CAD build for the part. Positions are in the model's coordinates, mm. Face numbers are marked on the shaded views. A direction names the side the tool comes from. Give positions to 0.01 mm unless a question says otherwise; leave off trailing zeros. Write each loop counter-clockwise with the first axis right and the second up, starting at its lowest first coordinate (ties: lowest second). Pieces come first, ordered by that corner, then holes. Notation, with made-up numbers: (25, 65) - (60, 65) arc R21 cw to (60, 100) - close; hole circle Ø5 at (-23, 40). An arc over 180 degrees is marked (long way). Answer as a JSON object with one key per item and string values.
from build123d import *

# Parameters (mm, degrees)
F0_R     = 19.05
F0_R_2   = 3.81
F0_R_3   = 5.4991
F1_DEPTH = 6.35
F0_R_4   = 2.7305
F2_DEPTH = 19.05
F4_DEPTH = 2


# Not quite as in the source:
# - a fillet or chamfer that OpenCascade refuses, or shapes differently, is made with other operations: its cross-section is extruded or revolved along the edge and cut away or added


with BuildPart() as f1:
    # F0 (on Top) → F1 (new body)
    with BuildSketch(Plane.XY):
        Circle(F0_R)
        with Locations((-9.6237072996, -5.55625)):
            Circle(F0_R_2, mode=Mode.SUBTRACT)
        with Locations((9.6237072996, -5.55625)):
            Circle(F0_R_2, mode=Mode.SUBTRACT)
        Circle(F0_R_3, mode=Mode.SUBTRACT)
        with Locations((0, 11.1125)):
            Circle(F0_R_2, mode=Mode.SUBTRACT)
    extrude(amount=F1_DEPTH)

    # F0 (on Top) → F2 (join)
    with BuildSketch(Plane.XY):
        Circle(F0_R_3)
        Circle(F0_R_4, mode=Mode.SUBTRACT)
    extrude(amount=F2_DEPTH)

    # F3 (on face) → F4 (cut)
    with BuildSketch(Plane.XY.offset(19.05)):
        with BuildLine():
            Line((1, 2.5407932324), (1, 5.4074116553))
            ThreePointArc((1, 5.4074116553), (0, 5.4991), (-1, 5.4074116553))
            Line((-1, 5.4074116553), (-1, 2.5407932324))
            ThreePointArc((-1, 2.5407932324), (0, 2.7305), (1, 2.5407932324))
        make_face()
        with BuildLine():
            Line((1, -5.4074116553), (1, -2.5407932324))
            ThreePointArc((1, -2.5407932324), (0, -2.7305), (-1, -2.5407932324))
            Line((-1, -2.5407932324), (-1, -5.4074116553))
            ThreePointArc((-1, -5.4074116553), (0, -5.4991), (1, -5.4074116553))
        make_face()
    extrude(amount=-F4_DEPTH, mode=Mode.SUBTRACT)

    # F5: chamfer of 4.445 on 1 edges, made by hand

    # F5_s1 → F5_t2 (revolve, cut)
    with BuildSketch(Plane.XZ):
        Polygon((19.05, 4.445), (14.605, 0), (19.05, 0), align=None)
    revolve(axis=Axis((0, 0, 0), (0, 0, 1)), mode=Mode.SUBTRACT)


solid = f1.part
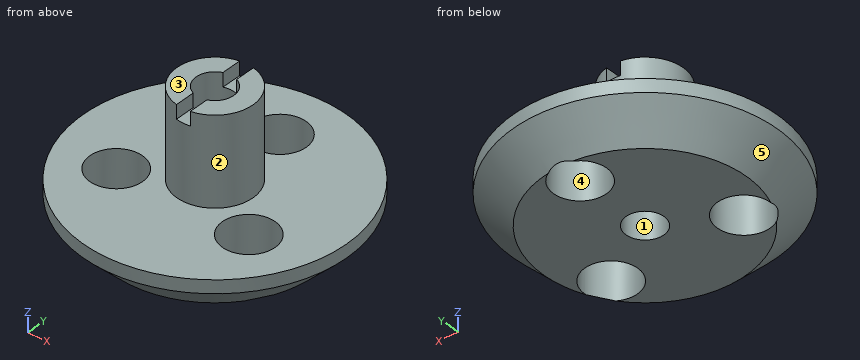
(1) Pull direction X, two halves, no side cores. Call the marked faces 3, 4 and 5: pulls with the +X half, pulls with the -X half, needs draft (parallel to the pull), parting line crosses it, or undercut.
Answer key:
{"face 3": "needs draft", "face 4": "undercut", "face 5": "parting line crosses it"}
(2) Flat gauge pins, fed straight in: P1, Ø8, axis at x = -15, y = -11, coming from the +Z side; P2, Ø1.6, axis at x = 0, y = -4.5, coming from the +Z side; P3, Ø1, axis at y = -4.5, z = 17.5, coming from the -X side. Where does each tip first touch, or does it go through?
Answer key:
{"P1": "stops at z = 6.35", "P2": "stops at z = 17.05", "P3": "stops at x = -3.77"}
(3) Probe L1, parallel to Y at x = 1.5, z = 3.5; L2, parallel to X at y = 0, z = 10; L3, parallel to X at y = -6.5, z = 2.5. List the from-to ranges inside material, lowest first. Write a range as [from, to].
Answer key:
{"L1": "y = [-18.04, -2.28], [2.28, 7.61], [14.61, 18.04]", "L2": "x = [-5.5, -2.73], [2.73, 5.5]", "L3": "x = [-15.82, -13.31], [-5.93, 5.93], [13.31, 15.82]"}
(4) 3-axis set-ups, long thin cutter, end or side, ignore diameter. For the marked faces 1 and 2: which of +Z, -Z, +X, -X, +Y, -Y reach the whole face in a straight line?
Answer key:
{"face 1": "+Z, -Z", "face 2": "+Z"}
(5) Saw through at C-C, the plane z = 15.25. Give the cut face in (x, y), and give its area (3 significant figures).
Answer key:
{"outline": "circle Ø11 at (0, 0); hole circle Ø5.46 at (0, 0)", "area": "71.6 mm²"}
(6) Saw through at B-B, the plane x = 0. State how many separate pieces and enclosed holes the cut face has, and give its area (3 significant figures).
Answer key:
{"separate pieces": "3", "enclosed holes": "0", "area": "198 mm²"}
